Could you check a few things on this model? Use its own coordinates, in mm. A direction names the side the tool comes from. Round coordinates to 2 decimals unless told otherwise and drop trailing zeros. Loops run counter-clockwise (first coordinate to the right, second up) from the corner with the lowest first, then second, coordinate; pieces in that order, holes last. Notation, with made-up numbers: (87.25, -35) - (106.25, -35) arc R30 ccw to (106.25, -7) - close; hole circle Ø10 at (64, -22.75). An arc over 180 degrees is marked (long way). Use one line per item in the form item = value.
```python
from build123d import *

# Parameters (mm, degrees)
F0_W      = 15.83
F0_H      = 7.87
F1_DEPTH  = 3.21
F2_W      = 13.03
F2_H      = 4.67
F3_DEPTH  = 1.75
F4_R      = 1.505
F4_R_2    = 0.565
F5_DEPTH  = 1.75
F6_W      = 7.66
F6_H      = 1.57
F7_DEPTH  = 9.58
F8_R      = 1.55
F9_DEPTH  = 9.58
F10_R     = 1.385
F11_DEPTH = 4.35


with BuildPart() as f1:
    # F0 (on Front) → F1 (new body)
    with BuildSketch(Plane.XZ):
        with Locations((7.915, 3.935)):
            Rectangle(F0_W, F0_H)
    extrude(amount=F1_DEPTH)

    # F2 (on face) → F3 (cut)
    with BuildSketch(Plane(origin=(0, 0, 0), x_dir=(-1, 0, 0), z_dir=(0, 1, 0))):
        with Locations((-7.915, 3.935)):
            Rectangle(F2_W, F2_H)
    extrude(amount=-F3_DEPTH, mode=Mode.SUBTRACT)

    # F4 (on face) → F5 (join, through all)
    with BuildSketch(Plane(origin=(0, -1.75, 0), x_dir=(-1, 0, 0), z_dir=(0, 1, 0))):
        with Locations((-7.915, 3.935)):
            Circle(F4_R)
        with Locations((-7.915, 3.935)):
            Circle(F4_R_2, mode=Mode.SUBTRACT)
    extrude(amount=F5_DEPTH)

    # F6 (on face) → F7 (join)
    with BuildSketch(Plane.XZ.offset(3.21)):
        with Locations((8, 7.085)):
            Rectangle(F6_W, F6_H)
    extrude(amount=F7_DEPTH)

    # F8 (on face) → F9 (join, through all)
    with BuildSketch(Plane.XZ.offset(12.79)):
        with Locations((8, 6.3)):
            Circle(F8_R)
    extrude(amount=-F9_DEPTH)

    # F10 (on face) → F11 (join)
    with BuildSketch(Plane.XZ.offset(12.79)):
        with Locations((8, 6.3)):
            Circle(F10_R)
    extrude(amount=F11_DEPTH)


solid = f1.part
```
1. For P1, Ø1.8, axis at x = 10.5, y = -6, coming from the -Z side; P2, Ø0.9, axis at x = 7.915, z = 3.935, coming from the -Y side; P3, Ø1.3, axis at y = -6, z = 7.5, coming from the -X side; P4, Ø2, axis at x = 13, y = -6.5, coming from the +Z side, each with a flat end and sliding along its axis, tell me the tip position at first contact or that it passes through.
Solution:
P1 = 6.3
P2 = -3.21
P3 = 4.17
P4 = through
2. If we section it at C-C, the plane x = 8: Write out the boundary of the cut face in (y, z) (3 decimals).
Solution:
outline = (-17.14, 4.915) - (-12.79, 4.915) - (-12.79, 4.75) - (-3.21, 4.75) - (-3.21, 0) - (0, 0) - (0, 1.6) - (-1.75, 1.6) - (-1.75, 2.432) - (0, 2.432) - (0, 3.376) - (-1.75, 3.376) - (-1.75, 4.494) - (0, 4.494) - (0, 5.438) - (-1.75, 5.438) - (-1.75, 6.27) - (0, 6.27) - (0, 7.87) - (-12.79, 7.87) - (-12.79, 7.685) - (-17.14, 7.685) - close
3. Please list where these lines run through material, in increasing order: line 1 along Y through (x, z) = (10.5, 2.5); line 2 along Y through (x, z) = (9.75, 7.25); line 3 along Z through (x, y) = (11.25, -11.25).
Solution:
line_1 = -3.21 to -1.75
line_2 = -12.79 to 0
line_3 = 6.3 to 7.87
4. We'd pull the mould along X, two halves only. Please class faces 1 (the face through (15.83, -2, 4)), 2 (the face through (7.376, -0.887, 4.105)), 3 (the face through (8, -5, 7.87)): +X half, -X half, draft (parallel to the pull), parting line (faces both ways), or undercut.
Solution:
face_1 = +X half
face_2 = undercut
face_3 = draft
5. If we section it at B-B, the plane z = 2: Write out the boundary of the cut face in (x, y).
Solution:
outline = (0, -3.21) - (15.83, -3.21) - (15.83, 0) - (14.43, 0) - (14.43, -1.75) - (1.4, -1.75) - (1.4, 0) - (0, 0) - close
6. On a 3-axis mill with a long thin cutter (end or side, diameter ignored), from which of +Z, -Z, +X, -X, +Y, -Y can I reach the whole of each face in a straight line? I mean faces 4 (the face through (8, -1, 1.6)), 5 (the face through (5, -8, 6.3)), 6 (the face through (11, -8, 6.3)), 7 (the face through (8, 0, 1)), 8 (the face through (7.97, -8.07, 4.75)). Say none if no direction works.
Solution:
face_4 = +Y
face_5 = -Z, -X, -Y
face_6 = -Z, +X, -Y
face_7 = +Z, -Z, +X, -X, +Y
face_8 = -Z, -Y
7. If we section it at A-A, the plane y = -1.25: Write out the boundary of the cut face in (x, z) (3 decimals).
Solution:
outline = (0, 0) - (15.83, 0) - (15.83, 7.87) - (0, 7.87) - close; circle Ø3.01 at (7.915, 3.935); hole (1.4, 1.6) - (14.43, 1.6) - (14.43, 6.27) - (1.4, 6.27) - close; hole circle Ø1.13 at (7.915, 3.935)
8. If we section it at D-D, the plane y = -11.5: Write out the boundary of the cut face in (x, z).
Solution:
outline = (4.17, 6.3) - (6.45, 6.3) arc R1.55 ccw to (9.55, 6.3) - (11.83, 6.3) - (11.83, 7.87) - (4.17, 7.87) - close
